```python
from build123d import *

# Parameters (mm, degrees)
F0_W     = 97.028
F0_H     = 29.2862
F1_DEPTH = 63.5
F2_R     = 3.2385
F3_DEPTH = 50.8
F5_DEPTH = 50.8


with BuildPart() as f1:
    # F0 (on Top) → F1 (new body)
    with BuildSketch(Plane.XY):
        with Locations((3.356052, -0.137089)):
            Rectangle(F0_W, F0_H)
    extrude(amount=F1_DEPTH)

    # F2 (on face) → F3 (cut)
    with BuildSketch(Plane.XZ.offset(14.780189)):
        with Locations((3.305252, 20.828)):
            Circle(F2_R)
    extrude(amount=-F3_DEPTH, mode=Mode.SUBTRACT)

    # F4 (on face) → F5 (cut)
    with BuildSketch(Plane.XZ.offset(14.780189)):
        Polygon((17.332412, 42.000698), (3.790186, 55.542924), (-5.854609, 45.898129), (-4.561452, 44.604972), (3.790186, 52.95661), (16.039255, 40.707541), align=None)
    extrude(amount=-F5_DEPTH, mode=Mode.SUBTRACT)


solid = f1.part
```
CAD build for the part. Positions are in the model's coordinates, mm. A direction names the side the tool comes from. Round coordinates to 2 decimals unless told otherwise and drop trailing zeros. Write each loop counter-clockwise with the first axis right and the second up, starting at its lowest first coordinate (ties: lowest second). Pieces come first, ordered by that corner, then holes. Notation, with made-up numbers: (24.25, -10.75) -> (45.25, -10.75) arc R13 cw to (45.25, 12.25) -> close; hole circle Ø10 at (34, 33.5). An arc over 180 degrees is marked (long way). Answer in a Markdown table with one row per item. Add a question column.
Item 1: Drop a flat-ended pin along its axis: pin 1 Ø5 at (x, z) = (3.31, 20.83) entering from +Y. Give the stop position or say it passes through.
Item 2: Which spindle directions (+Z, -Z, +X, -X, +Y, -Y) get a long thin tool onto all of the face, cutting with end or side? Do faces 4 (the face through (51.87, 0, 31)), 5 (the face through (-0.444, -0.342, 48.722)). Say none if no direction does.
Item 3: Saw through at A-A, the plane x = 13.5. Write the cut outline in (y, z).
Item 4: Drill centre lines: line 1 (X direction, y = 7.5, z = 51.5); line 2 (X direction, y = -0.5, z = 49.5); line 3 (Z direction, x = 4.5, y = -2.5). Where is each one in solid material? Low to high. Write a range as from..to.
Item 5: Mould opens along Z. For faces 1 (the face through (9.829, -0.342, 46.918)), 2 (the face through (3, 0, 0)), 3 (the face through (3, 14.506, 31)) say: pulls with the +Z half, pulls with the -Z half, needs draft (parallel to the pull), parting line crosses it, or undercut.
Findings below:
| question | item | result |
|---|---|---|
| 1 | pin 1 | passes through |
| 2 | face 4 | +Z, -Z, +X, +Y, -Y |
| 2 | face 5 | +Y, -Y |
| 3 | outline | (-14.78, 0) -> (14.51, 0) -> (14.51, 43.25) -> (-14.78, 43.25) -> close; (-14.78, 45.83) -> (14.51, 45.83) -> (14.51, 63.5) -> (-14.78, 63.5) -> close |
| 4 | line 1 | x = -45.16..-0.25, 2.33..5.25, 7.83..51.87 |
| 4 | line 2 | x = -45.16..-2.25, 0.33..7.25, 9.83..51.87 |
| 4 | line 3 | z = 0..17.82, 23.84..52.25, 54.83..63.5 |
| 5 | face 1 | undercut |
| 5 | face 2 | pulls with the -Z half |
| 5 | face 3 | needs draft |
